Read the model definition and answer for the solid it produces. Units are mm, in the model's axes. A direction names the side the tool comes from. Give positions to 0.01 mm unless a question says otherwise; leave off trailing zeros. Write each loop counter-clockwise with the first axis right and the second up, starting at its lowest first coordinate (ties: lowest second). Pieces come first, ordered by that corner, then holes. Notation, with made-up numbers: (38.25, 45) -> (84.25, 45) arc R20 cw to (84.25, 50) -> close; hole circle Ø8 at (-36.5, 61.5). An arc over 180 degrees is marked (long way). Answer as CSV lines item,"result". Start each with the question number.
1. The part is cut by section A-A, the plane z = 0. Determine the outline of the cut face in (x, y).
2. For a pull along Z with two mould halves and no side action, classify faces 3 (the flat face through (-0.99, 3.77, -1.74)), 4 (the cylindrical face through (-0.54, -7.4, 2.44)), 5 (the flat face through (-2, 0, 2)) as pulls with the +Z half, pulls with the -Z half, needs draft (parallel to the pull), parting line crosses it, or undercut.
3. Find the intervals of material crossed by line 1 (Z direction, x = 1.5, y = -10.25); line 2 (Y direction, x = -2.5, z = -2.5); line 3 (Z direction, x = 2.25, y = 3), in increasing order.
4. Given pin 1 (1 mm diameter, centred on y = -1, z = -2.5, fed in from +X); pin 2 (0.7 mm diameter, centred on y = 3.5, z = -0.5, fed in from -X); pin 3 (0.7 mm diameter, centred on y = 4, z = -0.5, fed in from +X), each flat-ended and moving along its own axis, determine where each tip first touches the part or whether it passes through.
5. The part is cut by section B-B, the plane y = -5. Determine the outline of the cut face in (x, z).
6. A tool of negligible diameter and unlimited length cuts with its end or side. For faces 1 (the cylindrical face through (-2.285, 2.32, -3.584)), 2 (the flat face through (-1.014, 3.768, 1.724)), from which of +Z, -Z, +X, -X, +Y, -Y can it reach the whole face along a straight path? Write none if from no direction.
7. The part is cut by section C-C, the plane y = 1.5. Determine the outline of the cut face in (x, z).
Autodesk Inventor part; units mm, degrees
ref_plane "YZ Plane" through (0, 0, 0) normal (1, 0, 0) x (0, 1, 0)
ref_plane "XZ Plane" through (0, 0, 0) normal (0, 1, 0) x (-1, 0, 0)
ref_plane "XY Plane" through (0, 0, 0) normal (0, 0, 1) x (1, 0, 0)
sketch "スケッチ1" plane through (0, 0, 0) normal (0, 1, 0) x (-1, 0, 0)
  circle A0 centre (0, 0) radius 4.25
  dimension "d0" = 8.5
extrude "押し出し1" add sketch "スケッチ1" along normal blind 5
sketch "スケッチ2" plane through (0, 0, 0) normal (0, -1, 0) x (1, 0, 0)
  circle A0 centre (0, 0) radius 2.5
  dimension "d3" = 5
extrude "押し出し2" add sketch "スケッチ2" along normal blind 15
fillet "フィレット1" radius 0.5 1 edges at (4.25, 5, 0)
fillet "フィレット1" radius 0.2 1 edges at (4.25, 0, 0)
sketch "スケッチ3" plane through (0, 5, 0) normal (0, 1, 0) x (1, 0, 0)
  line L0 (0, 2.3094) -> (-2, 1.1547)
  line L1 (-2, 1.1547) -> (-2, -1.1547)
  line L2 (-2, -1.1547) -> (0, -2.3094)
  line L3 (0, -2.3094) -> (2, -1.1547)
  line L4 (2, -1.1547) -> (2, 1.1547)
  line L5 (2, 1.1547) -> (0, 2.3094)
  line L6 (0, 2.3094) -> (0, -2.3094) construction
  circle A0 centre (0, 0) radius 2.3094 construction
  dimension "d12" = 4
extrude "押し出し3" cut sketch "スケッチ3" against normal blind 2.5
thread "ねじ2"
properties part number "M3-CapScrew"
Results found:
1,outline,"(-4.25, 0.2) arc R0.2 ccw to (-4.05, 0) -> (-2.5, 0) -> (-2.5, -15) -> (2.5, -15) -> (2.5, 0) -> (4.05, 0) arc R0.2 ccw to (4.25, 0.2) -> (4.25, 4.5) arc R0.5 ccw to (3.75, 5) -> (2, 5) -> (2, 2.5) -> (-2, 2.5) -> (-2, 5) -> (-3.75, 5) arc R0.5 ccw to (-4.25, 4.5) -> close"
2,face 3,"undercut"
2,face 4,"parting line crosses it"
2,face 5,"needs draft"
3,line 1,"z = -2 to 2"
3,line 2,"y = 0 to 5"
3,line 3,"z = -3.61 to 3.61"
4,pin 1,"stops at x = 1.5"
4,pin 2,"stops at x = -4.25"
4,pin 3,"stops at x = 4.25"
5,outline,"circle Ø5 at (0, 0)"
6,face 1,"+Y, -Y"
6,face 2,"+Y"
7,outline,"circle Ø8.5 at (0, 0)"
